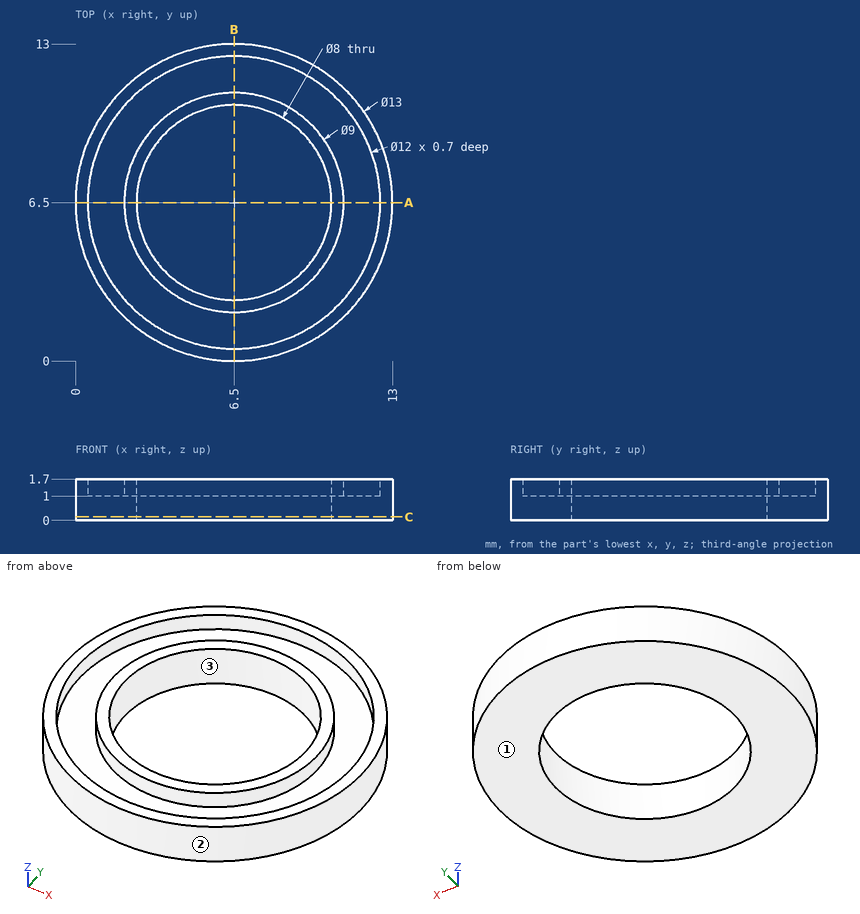
Geometry: see drawing. Coordinates: mm, zero at the bounding-box minimum. Coordinates: 2 decimals unless noted, no trailing zeros. Order: outer loops, then holes, each group sorted by start corner. A loop starts at its lowest first (then second) coordinate and runs counter-clockwise, first axis right, second up. Notation, with made-up numbers: M -9,11 L 46,11 A21 cw 46,17 Z; hole C 45,24.25 d8. An arc over 180 degrees is marked long. Answer as CSV lines item,"result".
1. Material intervals for line 1 (Y direction, x = 6.5, z = 1.5); line 2 (X direction, y = 3.25, z = 1.6); line 3 (Z direction, x = 7.25, y = 11), sorted ascending. Write a range as from..to.
Reported:
line 1,"0..0.5, 2..2.5, 10.5..11, 12.5..13"
line 2,"0.87..1.46, 3.39..4.17, 8.83..9.61, 11.54..12.13"
line 3,"0..1"
2. Pull-direction query (Y, two-part tool) for the marked faces 1, 2 and 3; classes: released by +Y, released by -Y, zero draft, split by the parting line, or undercut.
Reported:
face 1,"zero draft"
face 2,"split by the parting line"
face 3,"undercut"
3. Section A-A (y = 6.5). Return the cut outline in (x, z), then the cut area to 3 significant figures.
Reported:
outline,"M 0,0 L 2.5,0 L 2.5,1.7 L 2,1.7 L 2,1 L 0.5,1 L 0.5,1.7 L 0,1.7 Z; M 10.5,0 L 13,0 L 13,1.7 L 12.5,1.7 L 12.5,1 L 11,1 L 11,1.7 L 10.5,1.7 Z"
area,"6.40 mm2"
4. First-contact query: P1, Ø1, axis at y = 10.5, z = 1, coming from the -X side; P2, Ø7, axis at x = 6.5, y = 6.5, coming from the -Z side; P3, Ø1, axis at x = 11, z = 0.5, coming from the -Y side; P4, Ø1, axis at y = 7.5, z = 1.5, coming from the -X side. Flat tips, straight axial feed; report the tip coordinate or a pass-through.
Reported:
P1,"x = 1.02"
P2,"through"
P3,"y = 1.38"
P4,"x = 0.02"
5. Section C-C (z = 0.15). Return the cut outline in (x, y).
Reported:
outline,"C 6.5,6.5 d13; hole C 6.5,6.5 d8"
